For this review, take the finished solid that the model builds, in its own axes (mm). Round coordinates to 2 decimals unless told otherwise and drop trailing zeros. Answer as CSV lines item,"result". Start each with the question number.
Item 1: Take a section at A-A on z = -120.65. Count the separate pieces of the cut face and the enclosed holes in it, then the cut area to 3 significant figures.
Item 2: Mouldability with a two-part tool opening along Z and no side actions: class faces 1 (the flat face through (-2, 3, -136.525)), 2 (the flat face through (-136.525, 3, 2)), 3 (the cylindrical face through (-92.03, 3.22, 117.14)), 4 (the cylindrical face through (51.662, 3.219, -0.413)) as +Z half, -Z half, draft (parallel to the pull), parting line (faces both ways), or undercut.
Item 3: For pin 1 Ø8.5 at (x, z) = (-69.85, 120.65) entering from +Y, flat-tipped, find the tip position at first contact; note if it passes through.
Item 4: Wall thickness on probe 1 along X at (y, z) = (1.5, -120.65) (1 decimal); probe 2 along X at (y, z) = (2.5, 120.65) (1 decimal); probe 3 along X at (y, z) = (1.75, 0) (1 decimal): over which ranges is each line inside the solid? List them lowest first. Write a range as from..to.
```python
from build123d import *

# Parameters (mm, degrees)
SKETCH1_W           = 273.05
SKETCH1_H           = 273.05
SKETCH1_R           = 11.1125
BOSS_EXTRUDE1_DEPTH = 6.35
SKETCH2_R           = 4.7625
CUT_EXTRUDE1_DEPTH  = 194.179899964
SKETCH3_R           = 3.175
CUT_EXTRUDE4_DEPTH  = 194.179899964


with BuildPart() as part:
    # Sketch1 → Boss-Extrude1 (new body)
    with BuildSketch(Plane(origin=(0, 0, 0), x_dir=(1, 0, 0), z_dir=(0, 1, 0))):
        Rectangle(SKETCH1_W, SKETCH1_H)
        with Locations(Location((0, 0, 0), (0, 0, 270))):
            Circle(SKETCH1_R, mode=Mode.SUBTRACT)
    extrude(amount=BOSS_EXTRUDE1_DEPTH)

    # Sketch2 → Cut-Extrude1 (cut, through all)
    with BuildSketch(Plane(origin=(0, 6.35, 0), x_dir=(-1, 0, 0), z_dir=(0, 1, 0))):
        with Locations(Location((120.65, -120.65, 0), (0, 0, 90))):
            Circle(SKETCH2_R)
        with Locations(Location((120.65, 120.65, 0), (0, 0, 270))):
            Circle(SKETCH2_R)
        with Locations(Location((-120.65, -120.65, 0), (0, 0, 270))):
            Circle(SKETCH2_R)
        with Locations(Location((-120.65, 120.65, 0), (0, 0, 90))):
            Circle(SKETCH2_R)
        with Locations(Location((95.25, 120.65, 0), (0, 0, 90))):
            Circle(SKETCH2_R)
        with Locations(Location((69.85, 120.65, 0), (0, 0, 90))):
            Circle(SKETCH2_R)
        with Locations(Location((44.45, 120.65, 0), (0, 0, 90))):
            Circle(SKETCH2_R)
    extrude(amount=-CUT_EXTRUDE1_DEPTH, mode=Mode.SUBTRACT)

    # Sketch3 → Cut-Extrude4 (cut, through all)
    with BuildSketch(Plane(origin=(0, 6.35, 0), x_dir=(-1, 0, 0), z_dir=(0, 1, 0))):
        with Locations(Location((49.022, -28.194, 0), (0, 0, 90))):
            Circle(SKETCH3_R)
        with Locations(Location((49.022, 28.446, 0), (0, 0, 90))):
            Circle(SKETCH3_R)
        with Locations(Location((-48.514, 0, 0), (0, 0, 90))):
            Circle(SKETCH3_R)
    extrude(amount=-CUT_EXTRUDE4_DEPTH, mode=Mode.SUBTRACT)


solid = part.part
```
Output values:
1,separate pieces,"3"
1,enclosed holes,"0"
1,area,"1,610 mm^2"
2,face 1,"-Z half"
2,face 2,"draft"
2,face 3,"undercut"
2,face 4,"undercut"
3,pin 1,"passes through"
4,probe 1,"x = -136.5..-125.4, -115.9..115.9, 125.4..136.5"
4,probe 2,"x = -136.5..-125.4, -115.9..-100, -90.5..-74.6, -65.1..-49.2, -39.7..115.9, 125.4..136.5"
4,probe 3,"x = -136.5..-11.1, 11.1..45.3, 51.7..136.5"
